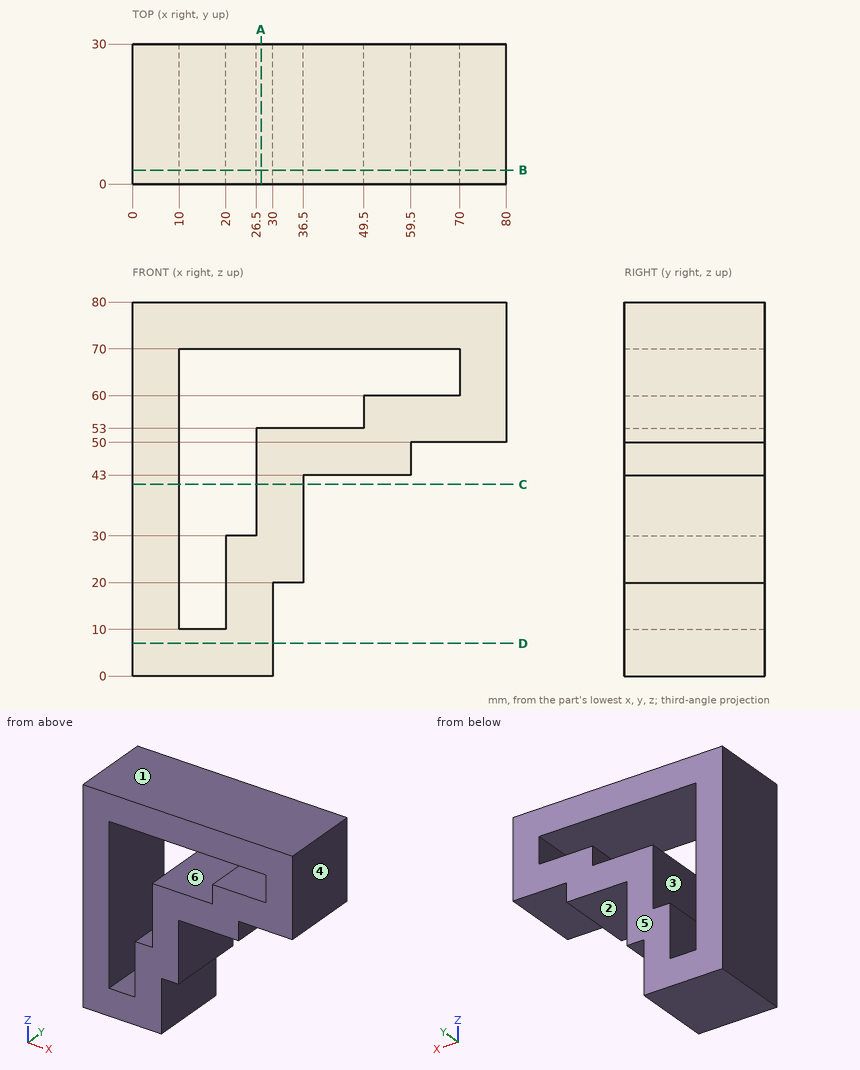
Geometry check sheet. Reference: drawing and pictorial views, mm from the part's lowest x, y, z. A direction names the side the tool comes from. Give positions to 0.01 mm unless a question says otherwise; leave off trailing zeros. Write each loop counter-clockwise with the first axis right and the second up, starting at its lowest first coordinate (ties: lowest second). Pieces come first, ordered by that corner, then holes. Notation, with made-up numbers: M 56.5,15 L 93.5,15 A32 ccw 93.5,43 Z; hole C 86.5,-5 d5. An arc over 180 degrees is marked long. Use CSV: the item, a comma, the result in double quotes.
1) Cross-section at D-D (z = 7). Enter the section's corners in (x, y), plus the area to 3 significant figures.
Final values:
outline,"M 0,0 L 30,0 L 30,30 L 0,30 Z"
area,"900 mm²"
2) Access from +Z, -Z, +X, -X, +Y, -Y to the whole of each face (thin tool, end or side, straight path). Record for the marked faces 1, 2 and 3.
Final values:
face 1,"+Z, +X, -X, +Y, -Y"
face 2,"-Z, +X, +Y, -Y"
face 3,"+Y, -Y"
3) Material ranges on line 1 along Z through (x, y) = (47.5, 18.5); line 2 along Z through (x, y) = (35, 2); line 3 along X through (y, z) = (2.5, 19), recorded low to high.
Final values:
line 1,"43 to 53, 70 to 80"
line 2,"20 to 53, 70 to 80"
line 3,"0 to 10, 20 to 30"
4) Cross-section at C-C (z = 41). Enter the section's corners in (x, y).
Final values:
outline,"M 0,0 L 10,0 L 10,30 L 0,30 Z; M 26.5,0 L 36.5,0 L 36.5,30 L 26.5,30 Z"
5) Cross-section at A-A (x = 27.5). Enter the section's corners in (y, z).
Final values:
outline,"M 0,0 L 30,0 L 30,53 L 0,53 Z; M 0,70 L 30,70 L 30,80 L 0,80 Z"
6) Go/stop test with flat-tipped pins: pin 1 Ø5.5 at (y, z) = (14.5, 45) entering from +X; pin 2 Ø5 at (x, y) = (33.5, 18) entering from -Z; pin 3 Ø10 at (x, y) = (70, 12) entering from -Z; pin 4 Ø2 at (x, z) = (57.5, 60.5) entering from +Y. Record where each tip stops, or that it passes through.
Final values:
pin 1,"x = 59.5"
pin 2,"z = 20"
pin 3,"z = 50"
pin 4,"y = 30"
7) Release check for a two-part mould opening along X. For the marked faces 4, 5 and 6 record: released by +X, released by -X, zero draft, split by the parting line, or undercut.
Final values:
face 4,"released by +X"
face 5,"zero draft"
face 6,"undercut"
8) Cross-section at B-B (y = 3). Enter the section's corners in (x, z).
Final values:
outline,"M 0,0 L 30,0 L 30,20 L 36.5,20 L 36.5,43 L 59.5,43 L 59.5,50 L 80,50 L 80,80 L 0,80 Z; hole M 10,10 L 20,10 L 20,30 L 26.5,30 L 26.5,53 L 49.5,53 L 49.5,60 L 70,60 L 70,70 L 10,70 Z"
